Source: CAD feature listing. Evaluate the final solid. Frame: model axes, mm. A direction names the side the tool comes from. Give positions to 0.01 mm unless a question says otherwise; leave off trailing zeros. Write each loop counter-clockwise with the first axis right and the second up, starting at its lowest first coordinate (ties: lowest second). Pieces come first, ordered by that corner, then holes. Notation, with made-up numbers: (61.25, 81.5) -> (76.25, 81.5) arc R31 ccw to (76.25, 107.5) -> close; hole circle Ø8 at (68.25, 75). An arc over 180 degrees is marked (long way). Answer as a JSON object with one key per item and string values. Group by question number.
Item 1: Access query for faces 1 (the face through (-13, -10, 5)), 2 (the face through (-4.315, 16, 5)), 3 (the face through (1, 17, 8)). Directions: +Z, -Z, +X, -X, +Y, -Y. A direction counts if a zero-diameter tool reaches every point of the face in a straight line with its end or side. Return the directions, or none.
Item 2: Pull-direction query (Z, two-part tool) for faces 4 (the face through (0, 6, 10)), 5 (the face through (-20, 0, 7)), 6 (the face through (1, -17, 6)), 7 (the face through (1, 17, 6)); classes: pulls with the +Z half, pulls with the -Z half, needs draft (parallel to the pull), parting line crosses it, or undercut.
Item 3: First-contact query: pin 1 Ø4 at (x, y) = (-27, 0) entering from +Z; pin 2 Ø1.5 at (x, z) = (-20, 2) entering from +Y; pin 3 Ø2.5 at (y, z) = (1, 8.5) entering from -X. Flat tips, straight axial feed; report the tip coordinate or a pass-through.
Item 4: Section query D-D on y = -13. Return the cut outline in (x, z).
Item 5: Section query C-C on z = 3.5. Return the cut outline in (x, y).
Item 6: Section query A-A on x = -6.5. Return the cut outline in (y, z).
Item 7: Ray query, probe 1 along Y at (x, z) = (27, 3.6); probe 2 along X at (y, z) = (1, 7.75); probe 3 along Y at (x, z) = (9, 0.75). Return the intervals inside material, ascending. Write a range as from..to.
Item 8: Section query B-B on y = 0. Return the cut outline in (x, z), plus the area to 3 significant figures.
from build123d import *

# Parameters (mm, degrees)
F0_W     = 10
F0_H     = 20
F0_W_2   = 28.184968
F0_R     = 1.5
F0_W_3   = 26.815032
F0_H_2   = 15
F1_DEPTH = 5
F2_W     = 40
F2_H     = 20
F2_W_2   = 10
F2_H_2   = 15
F3_DEPTH = 5
F4_W     = 10
F4_H     = 2
F5_DEPTH = 10
F6_W     = 30
F6_H     = 10
F7_DEPTH = 25
F8_R     = 5
F9_R     = 2.5


with BuildPart() as f1:
    # F0 (on Top) → F1 (new body)
    with BuildSketch(Plane.XY):
        with Locations((0.684968, 0)):
            Rectangle(F0_W, F0_H)
        with Locations((-18.407516, 0)):
            Rectangle(F0_W_2, F0_H)
        with Locations((-27, 0)):
            Circle(F0_R, mode=Mode.SUBTRACT)
        with Locations((19.092484, 0)):
            Rectangle(F0_W_3, F0_H)
        with Locations((27, 0)):
            Circle(F0_R, mode=Mode.SUBTRACT)
        with Locations((0.684968, 17.5)):
            Rectangle(F0_W, F0_H_2)
        with Locations((0.684968, -17.5)):
            Rectangle(F0_W, F0_H_2)
    extrude(amount=F1_DEPTH)

    # F2 (on face) → F3 (join)
    with BuildSketch(Plane.XY.offset(5)):
        Rectangle(F2_W, F2_H)
        with Locations((0.684968, 17.5)):
            Rectangle(F2_W_2, F2_H_2)
        with Locations((0.684968, -17.5)):
            Rectangle(F2_W_2, F2_H_2)
    extrude(amount=F3_DEPTH)

    # F4 (on face) → F5 (cut)
    with BuildSketch(Plane(origin=(-4.315032, 0, 0), x_dir=(0, -1, 0), z_dir=(-1, 0, 0))):
        with Locations((-17, 7)):
            Rectangle(F4_W, F4_H)
        with Locations((17, 7)):
            Rectangle(F4_W, F4_H)
    extrude(amount=-F5_DEPTH, mode=Mode.SUBTRACT)

    # F6 (on face) → F7 (cut)
    with BuildSketch(Plane.XY.offset(10)):
        Rectangle(F6_W, F6_H)
    extrude(amount=-F7_DEPTH, mode=Mode.SUBTRACT)

    # F8
    f8_edges = [f1.edges().sort_by_distance(p)[0] for p in [
        (-32.5, -10, 2.5),
        (-32.5, 10, 2.5),
        (32.5, 10, 2.5),
        (32.5, -10, 2.5),
    ]]
    fillet(f8_edges, radius=F8_R)

    # F9
    f9_edges = [f1.edges().sort_by_distance(p)[0] for p in [
        (-4.315032, -25, 5),
        (5.684968, -25, 5),
        (5.684968, 25, 5),
        (-4.315032, 25, 5),
    ]]
    fillet(f9_edges, radius=F9_R)


solid = f1.part
Worked answers:
{
 "1": {"face 1": "+Z, -Z, -X, -Y", "face 2": "+Z, -Z, -X, +Y", "face 3": "+X, -X"},
 "2": {"face 4": "pulls with the +Z half", "face 5": "needs draft", "face 6": "undercut", "face 7": "undercut"},
 "3": {"pin 1": "z = 5", "pin 2": "y = 10", "pin 3": "x = -20"},
 "4": {"outline": "(-4.32, 0) -> (5.68, 0) -> (5.68, 6) -> (-4.32, 6) -> close; (-4.32, 8) -> (5.68, 8) -> (5.68, 10) -> (-4.32, 10) -> close"},
 "5": {"outline": "(-32.5, -5) arc R5 ccw to (-27.5, -10) -> (-4.32, -10) -> (-4.32, -22.5) arc R2.5 ccw to (-1.82, -25) -> (3.18, -25) arc R2.5 ccw to (5.68, -22.5) -> (5.68, -10) -> (27.5, -10) arc R5 ccw to (32.5, -5) -> (32.5, 5) arc R5 ccw to (27.5, 10) -> (5.68, 10) -> (5.68, 22.5) arc R2.5 ccw to (3.18, 25) -> (-1.82, 25) arc R2.5 ccw to (-4.32, 22.5) -> (-4.32, 10) -> (-27.5, 10) arc R5 ccw to (-32.5, 5) -> close; hole circle Ø3 at (-27, 0); hole (-15, -5) -> (15, -5) -> (15, 5) -> (-15, 5) -> close; hole circle Ø3 at (27, 0)"},
 "6": {"outline": "(-10, 0) -> (-5, 0) -> (-5, 10) -> (-10, 10) -> close; (5, 0) -> (10, 0) -> (10, 10) -> (5, 10) -> close"},
 "7": {"probe 1": "-10..-1.5, 1.5..10", "probe 2": "-20..-15, 15..20", "probe 3": "-10..-5, 5..10"},
 "8": {"outline": "(-32.5, 0) -> (-28.5, 0) -> (-28.5, 5) -> (-32.5, 5) -> close; (-25.5, 0) -> (-15, 0) -> (-15, 10) -> (-20, 10) -> (-20, 5) -> (-25.5, 5) -> close; (15, 0) -> (25.5, 0) -> (25.5, 5) -> (20, 5) -> (20, 10) -> (15, 10) -> close; (28.5, 0) -> (32.5, 0) -> (32.5, 5) -> (28.5, 5) -> close", "area": "195 mm^2"}
}
